from build123d import *

# Parameters (mm, degrees)
EXTRUDE_1_DEPTH     = 16
FILLET_2_R          = 8
SKETCH_2_R          = 5
CUT_EXTRUDE_1_DEPTH = 2
SKETCH_3_R          = 3.5
CUT_EXTRUDE_2_DEPTH = 2


with BuildPart() as part:
    # 草图1 → 凸台-拉伸1 (new body)
    with BuildSketch(Plane(origin=(0, 0, 0), x_dir=(1, 0, 0), z_dir=(0, 1, 0))):
        Polygon((-8.6, 0), (8.6, 0), (17.8, 2.6), (17.8, 28.6), (19.6, 28.6), (19.6, 2.6), (19.6, 1.363414634), (8.6, -1.8), (-8.6, -1.8), (-13, 2.6), (-13, 28.6), (-11.2, 28.6), (-11.2, 2.6), align=None)
    extrude(amount=EXTRUDE_1_DEPTH)

    # 圆角2
    fillet_2_edges = [part.edges().sort_by_distance(p)[0] for p in [
        (18.7, 0, -28.6),
        (18.7, 16, -28.6),
        (-12.1, 0, -28.6),
        (-12.1, 16, -28.6),
    ]]
    fillet(fillet_2_edges, radius=FILLET_2_R - 0.0001)  # a hair under: the kernel refuses the full size

    # 草图2 → 切除-拉伸1 (cut)
    with BuildSketch(Plane.ZY.offset(13)):
        with Locations((-20.6, 8)):
            Circle(SKETCH_2_R)
    extrude(amount=-CUT_EXTRUDE_1_DEPTH, mode=Mode.SUBTRACT)

    # 草图3 → 切除-拉伸2 (cut)
    with BuildSketch(Plane(origin=(19.6, 0, 0), x_dir=(0, 0, -1), z_dir=(1, 0, 0))):
        with Locations((20.6, 8)):
            Circle(SKETCH_3_R)
    extrude(amount=-CUT_EXTRUDE_2_DEPTH, mode=Mode.SUBTRACT)


solid = part.part
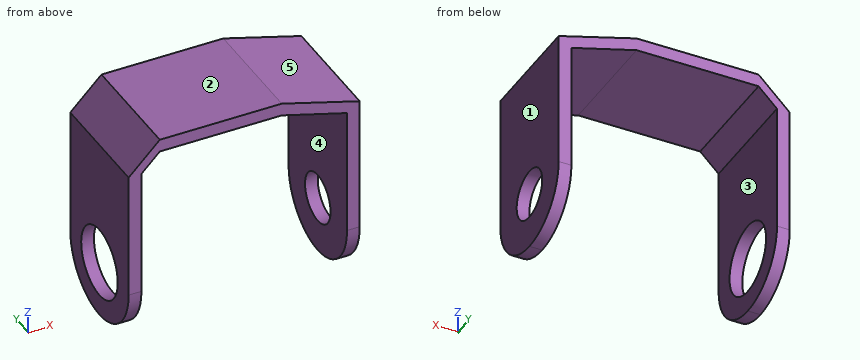
The listing builds one solid part. Answer for the finished solid, in the listing's coordinates (mm). Face numbers are marked on the shaded views. A direction names the side the tool comes from. Give positions to 0.01 mm unless a question says otherwise; leave off trailing zeros. Write each loop counter-clockwise with the first axis right and the second up, starting at its lowest first coordinate (ties: lowest second). Pieces come first, ordered by that corner, then holes.
1) Given P1, Ø8, axis at x = 10, z = -10.5, coming from the +Y side; P2, Ø5, axis at x = 11.5, y = 14, coming from the +Z side; P3, Ø5, axis at y = 9, z = -22, coming from the -X side; P4, Ø5, axis at x = -3, y = 4, coming from the -Z side, each flat-ended and moving along its own axis, determine where each tip first touches the part or whether it passes through.
2) Section A-A (z = -6.5) is taken. Write down the section's boundary in (x, y), and give its area (3 significant figures).
3) Section B-B (y = 1.5) is taken. Write down the section's boundary in (x, z), and give its area (3 significant figures).
4) A tool of negligible diameter and unlimited length cuts with its end or side. For the marked faces 4 and 5, from which of +Z, -Z, +X, -X, +Y, -Y can it reach the whole face along a straight path? Write none if from no direction.
5) Find the intervals of material crossed by L1, parallel to Y at x = 18.5, z = -20.6; L2, parallel to Y at x = -11.7, z = -20.6; L3, parallel to X at y = 2.75, z = -15.5, in increasing order.
6) Section C-C (x = -2) is taken. Write down the section's boundary in (y, z).
7) Section D-D (x = 12.5) is taken. Write down the section's boundary in (y, z), and give its area (3 significant figures).
8) For a pull along X with two mould halves and no side action, classify the marked faces 1, 2 and 3 as pulls with the +X half, pulls with the -X half, needs draft (parallel to the pull), parting line crosses it, or undercut.
Response:
1. P1: passes through
1. P2: stops at z = 1.68
1. P3: stops at x = 17.8
1. P4: stops at z = 0
2. outline: (-13, 0) - (-11.2, 0) - (-11.2, 16) - (-13, 16) - close; (17.8, 0) - (19.6, 0) - (19.6, 16) - (17.8, 16) - close
2. area: 57.6 mm2
3. outline: (-13, -25.26) - (-11.2, -25.26) - (-11.2, -2.6) - (-8.6, 0) - (8.6, 0) - (17.8, -2.6) - (17.8, -25.26) - (19.6, -25.26) - (19.6, -1.36) - (8.6, 1.8) - (-8.6, 1.8) - (-13, -2.6) - close
3. area: 138 mm2
4. face 4: -Z, +Y, -Y
4. face 5: +Z, +X, +Y, -Y
5. L1: y = 0 to 4.5, 11.5 to 16
5. L2: y = 0 to 3, 13 to 16
5. L3: x = -13 to -11.2, 17.8 to 19.6
6. outline: (0, 0) - (16, 0) - (16, 1.8) - (0, 1.8) - close
7. outline: (0, -1.1) - (16, -1.1) - (16, 0.68) - (0, 0.68) - close
7. area: 28.5 mm2
8. face 1: pulls with the +X half
8. face 2: needs draft
8. face 3: undercut
